Autodesk Inventor part; units mm, degrees
ref_plane "YZ Plane" through (0, 0, 0) normal (1, 0, 0) x (0, 1, 0)
ref_plane "XZ Plane" through (0, 0, 0) normal (0, 1, 0) x (-1, 0, 0)
ref_plane "XY Plane" through (0, 0, 0) normal (0, 0, 1) x (1, 0, 0)
sketch "Sketch1" plane through (0, 0, 0) normal (0, 1, 0) x (-1, 0, 0)
  line L0 (0, 0) -> (26.416, 0)
  line L1 (26.416, 0) -> (26.416, -26.416)
  line L2 (26.416, -26.416) -> (0, -26.416)
  line L3 (0, -26.416) -> (0, 0)
  line L4 (0, -13.208) -> (17.9832, -13.208)
  line L5 (0, -13.208) -> (17.9832, -13.208) construction
  circle A0 centre (17.9832, -13.208) radius 13.335
  point P0 (16.1472, 0)
  point P1 (16.1472, -26.416)
  dimension "d0" = 26.416
  dimension "d1" = 26.416
  dimension "d2" = 17.9832
  dimension "d3" = 0
  dimension "d4" = 26.67
extrude "Extrusion1" add sketch "Sketch1" along normal blind 12.7 contours L0 A0 L4 L3 | L4 A0 L2 L3
sketch "Sketch2" plane through (0, 0, 0) normal (1, 0, 0) x (0, 0, -1)
  line L0 (0, 12.7) -> (26.416, 12.7)
  line L1 (13.208, 12.7) -> (13.208, 6.35)
  line L2 (13.208, 12.7) -> (19.558, 12.7) construction
  line L3 (13.208, 6.35) -> (21.1328, 6.35)
  line L4 (13.208, 6.35) -> (21.1328, 6.35) construction
  line L5 (13.208, 6.35) -> (5.2832, 6.35)
  line L6 (13.208, 6.35) -> (21.1328, 6.35) construction
  point P0 (0, 0)
  dimension "d7" = 6.35
  dimension "d8" = 90
  dimension "d9" = 7.9248
  dimension "d10" = 0
  dimension "d11" = 7.9248
  dimension "d12" = 180
hole "Hole1" at (0, 6.35, -5.2832) at (0, 6.35, -21.1328) direction (-1, 0, 0) diameter 4.4958 depth 35
fillet "Fillet1" radius 3.175 2 edges at (0, 12.7, -13.208) (0, 0, -13.208)
sketch "Sketch3" plane through (0, 3.175, -26.416) normal (1, 0, 0) x (0, 0, -1)
  line L0 (-26.416, 9.525) -> (0, 9.525)
  line L1 (-26.416, -3.175) -> (0, -3.175)
  line L2 (-26.416, 9.525) -> (-25.146, 9.525)
  line L3 (-25.146, 9.525) -> (-25.146, -3.175)
  line L4 (-25.146, -3.175) -> (-26.416, -3.175)
  line L5 (-26.416, -3.175) -> (-26.416, 9.525)
  line L6 (0, -3.175) -> (0, 9.525)
  line L7 (0, 9.525) -> (-1.27, 9.525)
  line L8 (-1.27, 9.525) -> (-1.27, -3.175)
  line L9 (-1.27, -3.175) -> (0, -3.175)
  line L10 (0, -3.175) -> (0, 9.525)
  point P0 (-1.27, 9.525)
  point P1 (-1.27, -3.175)
  dimension "d21" = 1.27
  dimension "d22" = 1.27
extrude "Extrusion2" cut sketch "Sketch3" against normal blind 25.4 contours L0 L3 L1 L5 | L0 L6 L1 L8
properties part number "CatchHolderNut"
Input: part model. Units: mm. Frame: model coordinates. Coordinates: 2 decimals unless noted, no trailing zeros. Order: outer loops, then holes, each group sorted by start corner. A loop starts at its lowest first (then second) coordinate and runs counter-clockwise, first axis right, second up. Notation, with made-up numbers: (24.5, 77.25) - (55.5, 77.25) arc R14 ccw to (55.5, 82.25) - close; hole circle Ø11 at (-37.5, -6). An arc over 180 degrees is marked (long way). Return JSON: item names as keys, results as strings.
Q1. Draft query along Y for faces 1 (the flat face through (-4, 0, -13)), 2 (the flat face through (-6, 6, -25.146)), 3 (the cylindrical face through (-3.706, 6.251, -3.037)). Return one class per face: +Y half, -Y half, draft (parallel to the pull), parting line (faces both ways), or undercut.
The answers:
{"face 1": "-Y half", "face 2": "draft", "face 3": "undercut"}
Q2. First-contact query: pin 1 (2 mm diameter, centred on y = 11, z = -10.5, fed in from +X). Flat tip, straight axial feed; report the tip coordinate or a pass-through.
The answers:
{"pin 1": "stops at x = -0.04"}
Q3. Cut plane A-A (x = -5.5). Return loops of the section in (y, z).
The answers:
{"outline": "(0, -25.15) - (12.7, -25.15) - (12.7, -17.9) - (0, -17.9) - close; (0, -8.52) - (12.7, -8.52) - (12.7, -1.27) - (0, -1.27) - close; hole circle Ø4.5 at (6.35, -21.13); hole circle Ø4.5 at (6.35, -5.28)"}
Q4. Ray query, probe 1 along Z at (x, y) = (-3, 7.5); probe 2 along Z at (x, y) = (-6.75, 6.35); probe 3 along Z at (x, y) = (-7, 10.75). Return the intervals inside material, ascending.
The answers:
{"probe 1": "z = -25.15 to -23.06, -19.2 to -7.21, -3.35 to -1.27", "probe 2": "z = -25.15 to -23.38, -3.04 to -1.27", "probe 3": "z = -25.15 to -20.77, -5.65 to -1.27"}
Q5. Cut plane D-D (x = -3.75). Return loops of the section in (y, z).
The answers:
{"outline": "(0, -25.15) - (12.7, -25.15) - (12.7, -1.27) - (0, -1.27) - close; hole circle Ø4.5 at (6.35, -21.13); hole circle Ø4.5 at (6.35, -5.28)"}
Q6. Cut plane B-B (y = 7.5). Return loops of the section in (x, z) (3 decimals).
The answers:
{"outline": "(-12.041, -25.146) - (0, -25.146) - (0, -23.064) - (-9.001, -23.064) arc R13.335 cw to start; (-12.041, -1.27) arc R13.335 cw to (-9.001, -3.352) - (0, -3.352) - (0, -1.27) - close; (-6.071, -19.201) - (0, -19.201) - (0, -7.215) - (-6.071, -7.215) arc R13.335 cw to start"}
Q7. Cut plane C-C (x = -8). Return loops of the section in (y, z), then the cut area to 3 significant figures.
The answers:
{"outline": "(0, -25.15) - (12.7, -25.15) - (12.7, -22.05) - (8.4, -22.05) arc R2.25 cw to (4.3, -22.05) - (0, -22.05) - close; (0, -4.37) - (4.3, -4.37) arc R2.25 cw to (8.4, -4.37) - (12.7, -4.37) - (12.7, -1.27) - (0, -1.27) - close", "area": "70.8 mm2"}
